The figure shows three views and two pictorial views of one solid part (mm, origin at its lowest corner). Answer the questions. A direction names the side the tool comes from. Coordinates: 2 decimals unless noted, no trailing zeros. Loops run counter-clockwise (first coordinate to the right, second up) from the corner with the lowest first, then second, coordinate; pieces in that order, holes last. Notation, with made-up numbers: M -32.5,-19 L 5.5,-19 A10 ccw 5.5,-14 Z; hole C -38,77.5 d11. An arc over 180 degrees is marked long. Return JSON: item names as keys, results as strings. Group by question number.
1. Section C-C (x = 7) is taken. Write down the section's boundary in (y, z), then the cut area to 3 significant figures.
2. Section D-D (y = 4.75) is taken. Write down the section's boundary in (x, z).
3. Section A-A (y = 11.5) is taken. Write down the section's boundary in (x, z) (3 decimals).
4. Which of the six approach directions +Z, -Z, +X, -X, +Y, -Y give full straight-line access (tool end or side, diameter ignored) to the marked faces 1 and 2?
5. The mould has two halves that part along X. Classify the marked faces 3, 4 and 5: pulls with the +X half, pulls with the -X half, needs draft (parallel to the pull), parting line crosses it, or undercut.
6. Given P1, Ø5, axis at x = 10.5, z = 6, coming from the +Y side, flat-ended and moving along its own axis, determine where the tip first touches the part or whether it passes through.
7. Section B-B (z = 9) is taken. Write down the section's boundary in (x, y).
8. Straight lines are drawn through the part: L1, parallel to X at y = 11.5, z = 0.6 (3 decimals); L2, parallel to X at y = 0.65, z = 9; L3, parallel to Z at x = 11, y = 14.75. For each, find the intervals that lie inside material, in ascending order. Write a range as from..to.
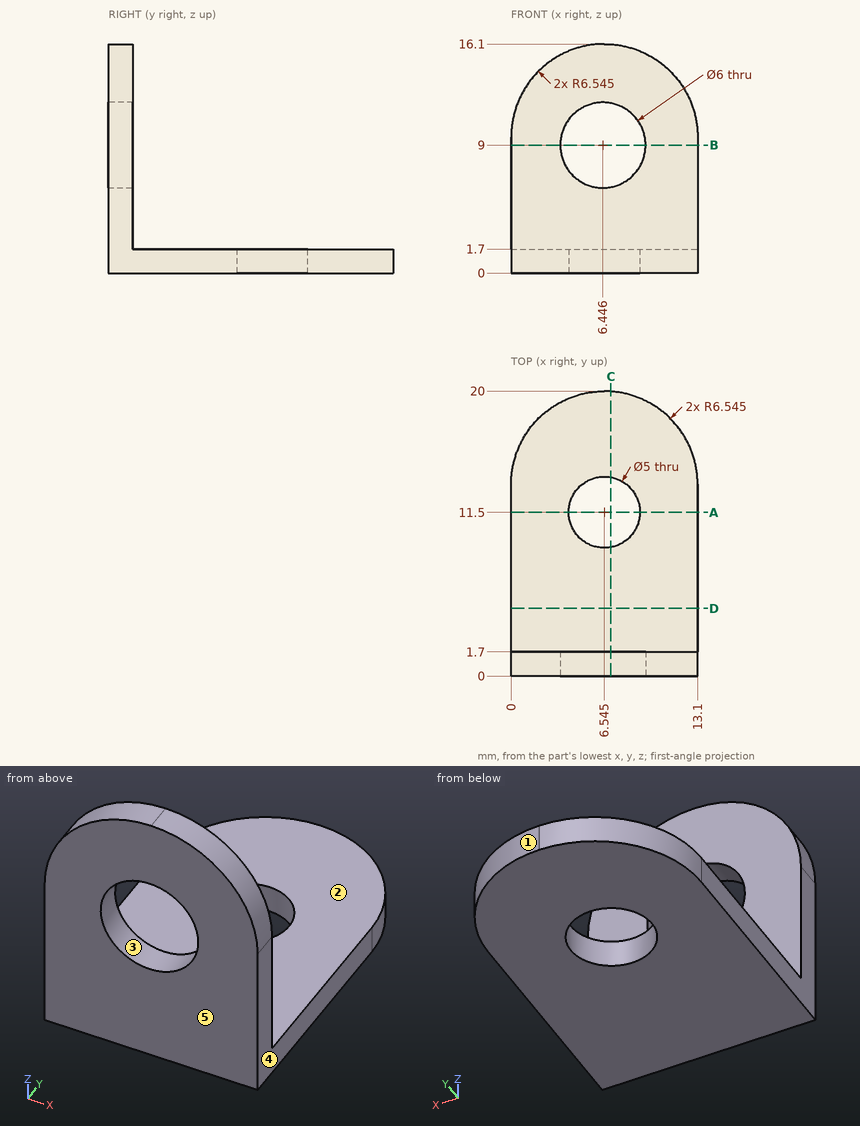
Worked out:
{
 "1": {"outline": "M 0,0 L 9.04,0 L 9.04,1.7 L 1.7,1.7 L 1.7,6.05 L 0,6.05 Z; M 0,11.95 L 1.7,11.95 L 1.7,16.08 L 0,16.08 Z; M 13.96,0 L 19.98,0 L 19.98,1.7 L 13.96,1.7 Z", "area": "40.0 mm^2"},
 "2": {"outline": "M 0,0 L 13.1,0 L 13.1,1.7 L 0,1.7 Z"},
 "3": {"outline": "M 0,0 L 4.045,0 L 4.045,1.7 L 0,1.7 Z; M 9.045,0 L 13.1,0 L 13.1,1.7 L 9.045,1.7 Z"},
 "4": {"face 1": "+Z, -Z, +X, +Y", "face 2": "+Z, +X, -X, +Y"},
 "5": {"face 3": "undercut", "face 4": "pulls with the +X half", "face 5": "needs draft"},
 "6": {"P1": "y = 1.7"},
 "7": {"outline": "M 0,0 L 3.45,0 L 3.45,1.7 L 0,1.7 Z; M 9.45,0 L 13.1,0 L 13.1,1.7 L 9.45,1.7 Z"},
 "8": {"L1": "0..4.045, 9.045..13.1", "L2": "0..3.45, 9.45..13.1", "L3": "0..1.7"}
}
